from build123d import *

# Parameters (mm, degrees)
SKETCH1_R           = 2.4892
SKETCH1_R_2         = 3.175
BOSS_EXTRUDE1_DEPTH = 3.175
FILLET1_R           = 12.7


with BuildPart() as part:
    # Sketch1 → Boss-Extrude1 (new body)
    with BuildSketch(Plane.XY):
        Polygon((0, 0), (50.8, 0), (50.8, -25.4), (26.67, -25.4), (26.67, -76.2), (0, -76.2), align=None)
        with Locations((44.45, -12.7)):
            Circle(SKETCH1_R, mode=Mode.SUBTRACT)
        with Locations((25.4, -12.7)):
            Circle(SKETCH1_R, mode=Mode.SUBTRACT)
        with Locations((6.35, -12.7)):
            Circle(SKETCH1_R_2, mode=Mode.SUBTRACT)
        with Locations((6.35, -38.1)):
            Circle(SKETCH1_R, mode=Mode.SUBTRACT)
        with Locations((6.35, -63.5)):
            Circle(SKETCH1_R, mode=Mode.SUBTRACT)
    extrude(amount=BOSS_EXTRUDE1_DEPTH)

    # Fillet1
    fillet1_edges = [part.edges().sort_by_distance(p)[0] for p in [
        (0, 0, 1.5875),
        (26.67, -25.4, 1.5875),
    ]]
    fillet(fillet1_edges, radius=FILLET1_R)


solid = part.part
Could you check a few things on this model? Use its own coordinates, in mm. A direction names the side the tool comes from. Give positions to 0.01 mm unless a question says otherwise; leave off trailing zeros. Order: outer loops, then holes, each group sorted by start corner. A loop starts at its lowest first (then second) coordinate and runs counter-clockwise, first axis right, second up.
1. Suppose I cut it at D-D (x = 6.35). List the corners of the cut face in (y, z) for me (3 decimals), plus the area to 3 significant figures.
2. Will these pins go through, and if not, where does the flat tip stop? P1, Ø6.5, axis at x = 6.35, y = -38.1, coming from the +Z side (3 decimals); P2, Ø12, axis at x = 35, y = -65, coming from the +Z side; P3, Ø1, axis at y = -62.5, z = 2.5, coming from the +X side; P4, Ø1, axis at x = 10, z = 1, coming from the +Y side.
3. Suppose I cut it at C-C (x = 25.4). List the corners of the cut face in (y, z) for me (3 decimals).
4. Suppose I cut it at A-A (y = -63.5). List the corners of the cut face in (x, z) for me (3 decimals).
5. Suppose I cut it at B-B (z = 1.1). List the corners of the cut face in (x, y) for me (3 decimals), plus the area to 3 significant figures.
6. We'd pull the mould along X, two halves only. Please class faces 1 (the cylindrical face through (46.75, -13.65, 1.57)), 2 (the cylindrical face through (30.49, -29.02, 1.61)), 3 (the flat face through (14, -76.2, 2)), 4 (the cylindrical face through (3.83, -14.63, 1.57)): pulls with the +X half, pulls with the -X half, needs draft (parallel to the pull), parting line crosses it, or undercut.
7. I need wall thicknesses on L1, parallel to X at y = -14.5, z = 0.2; L2, parallel to Y at x = 6.35, z = 1 (3 decimals); L3, parallel to Y at x = 4.5, z = 1.3. Which ranges of each line are inside material? Lowest first, please.
8. For faces 5 (the flat face through (26.67, -57, 2)), 6 (the flat face through (20, -38, 3.175)), which set-ups out of +Z, -Z, +X, -X, +Y, -Y let a thin tool reach every point of the face, with its end or its side?
Solved:
1. outline: (-76.2, 0) - (-65.989, 0) - (-65.989, 3.175) - (-76.2, 3.175) - close; (-61.011, 0) - (-40.589, 0) - (-40.589, 3.175) - (-61.011, 3.175) - close; (-35.611, 0) - (-15.875, 0) - (-15.875, 3.175) - (-35.611, 3.175) - close; (-9.525, 0) - (-1.701, 0) - (-1.701, 3.175) - (-9.525, 3.175) - close
1. area: 185 mm2
2. P1: stops at z = 3.175
2. P2: passes through
2. P3: stops at x = 26.67
2. P4: stops at y = -0.19
3. outline: (-76.2, 0) - (-15.189, 0) - (-15.189, 3.175) - (-76.2, 3.175) - close; (-10.211, 0) - (0, 0) - (0, 3.175) - (-10.211, 3.175) - close
4. outline: (0, 0) - (3.861, 0) - (3.861, 3.175) - (0, 3.175) - close; (8.839, 0) - (26.67, 0) - (26.67, 3.175) - (8.839, 3.175) - close
5. outline: (0, -76.2) - (26.67, -76.2) - (26.67, -38.1) arc R12.7 cw to (39.37, -25.4) - (50.8, -25.4) - (50.8, 0) - (12.7, 0) arc R12.7 ccw to (0, -12.7) - close; hole circle Ø6.35 at (6.35, -12.7); hole circle Ø4.978 at (6.35, -63.5); hole circle Ø4.978 at (6.35, -38.1); hole circle Ø4.978 at (25.4, -12.7); hole circle Ø4.978 at (44.45, -12.7)
5. area: 2,540 mm2
6. face 1: undercut
6. face 2: pulls with the +X half
6. face 3: needs draft
6. face 4: undercut
7. L1: x = 0 to 3.73, 8.97 to 23.68, 27.12 to 42.73, 46.17 to 50.8
7. L2: y = -76.2 to -65.989, -61.011 to -40.589, -35.611 to -15.875, -9.525 to -1.701
7. L3: y = -76.2 to -65.17, -61.83 to -39.77, -36.43 to -15.28, -10.12 to -3
8. face 5: +Z, -Z, +X, -Y
8. face 6: +Z, +X, -X, +Y, -Y
